```python
from build123d import *

# Parameters (mm, degrees)
SKETCH1_R                = 2.5
BOSS_EXTRUDE1_DEPTH      = 5
SKETCH3_W                = 20
SKETCH3_H                = 40
BOSS_EXTRUDE5_DEPTH      = 25
CUT_EXTRUDE2_DEPTH       = 75.20598847
CUT_EXTRUDE2_DEPTH_BACK  = 75.20598847
CUT_EXTRUDE_THIN13_DEPTH = 75.484252037
SKETCH8_W                = 5
SKETCH8_H                = 25
BOSS_EXTRUDE6_DEPTH      = 2
FILLET3_R                = 2
SKETCH9_W                = 5
SKETCH9_H                = 25
BOSS_EXTRUDE7_DEPTH      = 2
FILLET4_R                = 2
SKETCH11_R               = 4.5
CUT_EXTRUDE4_DEPTH       = 25
SKETCH12_R               = 6
SKETCH12_R_2             = 8
BOSS_EXTRUDE8_DEPTH      = 25
SKETCH13_R               = 2.5
CUT_EXTRUDE5_DEPTH       = 28
SKETCH14_R               = 4
CUT_EXTRUDE6_DEPTH       = 5
CUT_EXTRUDE7_DEPTH       = 18
CUT_EXTRUDE7_DEPTH_BACK  = 70
SKETCH15_R               = 2.5


with BuildPart() as part:
    # Sketch1 → Boss-Extrude1 (new body)
    with BuildSketch(Plane.XY):
        with BuildLine():
            Line((-33.639154819, 54.619565217), (6.360845181, 54.619565217))
            ThreePointArc((6.360845181, 54.619565217), (13.431912992, 51.690633029), (16.360845181, 44.619565217))
            Line((16.360845181, 44.619565217), (16.360845181, -5.380434783))
            ThreePointArc((16.360845181, -5.380434783), (13.431912992, -12.451502594), (6.360845181, -15.380434783))
            Line((6.360845181, -15.380434783), (-33.639154819, -15.380434783))
            ThreePointArc((-33.639154819, -15.380434783), (-40.710222631, -12.451502594), (-43.639154819, -5.380434783))
            Line((-43.639154819, -5.380434783), (-43.639154819, 44.619565217))
            ThreePointArc((-43.639154819, 44.619565217), (-40.710222631, 51.690633029), (-33.639154819, 54.619565217))
        make_face()
        with Locations((1.061250856, 48.159869042)):
            Circle(SKETCH1_R, mode=Mode.SUBTRACT)
        with Locations(Location((1.061250856, -9.840130958, 0), (0, 0, 180))):
            Circle(SKETCH1_R, mode=Mode.SUBTRACT)
        with Locations((-31.938749144, 19.159869042)):
            Circle(SKETCH1_R, mode=Mode.SUBTRACT)
    extrude(amount=BOSS_EXTRUDE1_DEPTH)

    # Sketch3 → Boss-Extrude5 (add)
    with BuildSketch(Plane.XY.offset(5)):
        Polygon((-24.438749144, 44.600432852), (-29.438749144, 44.600432852), (-29.438749144, 37.28199121), (-43.639154819, 37.28199121), (-43.639154819, 32.28199121), (-29.438749144, 32.28199121), (-29.438749144, 7.637328911), (-43.639154819, 7.637328911), (-43.639154819, 2.637328911), (-29.438749144, 2.637328911), (-29.438749144, -5.399567148), (-24.438749144, -5.399567148), (-24.438749144, -15.380434783), (-19.438749144, -15.380434783), (-19.438749144, -5.399567148), (-10.184597354, -5.399567148), (-10.184597354, -15.380434783), (-5.184597354, -15.380434783), (-5.184597354, -5.399567148), (0.561250856, -5.399567148), (0.561250856, 2.637328911), (14.825245568, 2.637328911), (14.825245568, 7.637328911), (0.561250856, 7.637328911), (0.561250856, 17.719700958), (14.825245568, 17.719700958), (14.825245568, 22.719700958), (0.561250856, 22.719700958), (0.561250856, 32.28199121), (14.825245568, 32.28199121), (14.825245568, 37.28199121), (0.561250856, 37.28199121), (0.561250856, 44.600432852), (-5.184597354, 44.600432852), (-5.184597354, 54.581300487), (-10.184597354, 54.581300487), (-10.184597354, 44.600432852), (-19.438749144, 44.600432852), (-19.438749144, 54.581300487), (-24.438749144, 54.581300487), align=None)
        with Locations((-14.438749144, 19.600432852)):
            Rectangle(SKETCH3_W, SKETCH3_H, mode=Mode.SUBTRACT)
    extrude(amount=BOSS_EXTRUDE5_DEPTH)

    # Sketch5 → Cut-Extrude2 (cut, two sides: drawn at the far end of the back side and taken through both)
    with BuildSketch(Plane.XZ.offset(-2.637328911).offset(-CUT_EXTRUDE2_DEPTH_BACK)):
        Polygon((-43.639154819, 30), (-43.639154819, 5), (-29.438749144, 30), align=None)
        Polygon((14.825245568, 30), (0.561250856, 30), (14.825245568, 5), align=None)
    extrude(amount=CUT_EXTRUDE2_DEPTH + CUT_EXTRUDE2_DEPTH_BACK, mode=Mode.SUBTRACT)

    # Sketch7 → Cut-Extrude-Thin13 (cut, through all)
    with BuildSketch(Plane.ZY.offset(24.438749144)):
        Polygon((30, 44.600432852), (5, 54.619565217), (8.72002984, 63.901880553), (33.72002984, 53.882748188), align=None)
        Polygon((5, -15.380434783), (30, -5.399567148), (33.707778838, -14.686782882), (8.707778838, -24.667650517), align=None)
    extrude(amount=-CUT_EXTRUDE_THIN13_DEPTH, mode=Mode.SUBTRACT)

    # Sketch8 → Boss-Extrude6 (add)
    with BuildSketch(Plane.XZ.offset(-39.600432852)):
        with Locations((-14.438749144, 17.5)):
            Rectangle(SKETCH8_W, SKETCH8_H)
    extrude(amount=BOSS_EXTRUDE6_DEPTH)

    # Fillet3
    fillet3_edges = [part.edges().sort_by_distance(p)[0] for p in [
        (-16.938749144, 37.600432852, 17.5),
        (-11.938749144, 37.600432852, 17.5),
    ]]
    fillet(fillet3_edges, radius=FILLET3_R - 0.0001)  # a hair under: the kernel refuses the full size

    # Sketch9 → Boss-Extrude7 (add)
    with BuildSketch(Plane(origin=(0, -0.399567148, 0), x_dir=(1, 0, 0), z_dir=(0, 1, 0))):
        with Locations((-14.690486301, -17.5)):
            Rectangle(SKETCH9_W, SKETCH9_H)
    extrude(amount=BOSS_EXTRUDE7_DEPTH)

    # Fillet4
    fillet4_edges = [part.edges().sort_by_distance(p)[0] for p in [
        (-12.190486301, 1.600432852, 17.5),
        (-17.190486301, 1.600432852, 17.5),
    ]]
    fillet(fillet4_edges, radius=FILLET4_R - 0.0001)  # a hair under: the kernel refuses the full size

    # Sketch11 → Cut-Extrude4 (cut)
    with BuildSketch(Plane.XY.offset(30)):
        with Locations((-31.938749144, 19.159869042)):
            Circle(SKETCH11_R)
    extrude(amount=-CUT_EXTRUDE4_DEPTH, mode=Mode.SUBTRACT)

    # Sketch12 → Boss-Extrude8 (add)
    with BuildSketch(Plane.XY.offset(5)):
        with Locations((1.061250856, 48.159869042)):
            Circle(SKETCH12_R)
        with Locations((1.061250856, -9.840130958)):
            Circle(SKETCH12_R)
        with Locations((-31.938749144, 19.159869042)):
            Circle(SKETCH12_R_2)
    extrude(amount=BOSS_EXTRUDE8_DEPTH)

    # Sketch13 → Cut-Extrude5 (cut)
    with BuildSketch(Plane(origin=(0, 0, 0), x_dir=(-1, 0, 0), z_dir=(0, 0, -1))):
        with Locations((31.938749144, 19.159869042)):
            Circle(SKETCH13_R)
        with Locations((-1.061250856, -9.840130958)):
            Circle(SKETCH13_R)
        with Locations((-1.061250856, 48.159869042)):
            Circle(SKETCH13_R)
    extrude(amount=-CUT_EXTRUDE5_DEPTH, mode=Mode.SUBTRACT)

    # Sketch14 → Cut-Extrude6 (cut)
    with BuildSketch(Plane.XY.offset(30)):
        with Locations((-31.938749144, 19.159869042)):
            Circle(SKETCH14_R)
        with Locations((1.061250856, 48.159869042)):
            Circle(SKETCH14_R)
        with Locations((1.061250856, -9.840130958)):
            Circle(SKETCH14_R)
    extrude(amount=-CUT_EXTRUDE6_DEPTH, mode=Mode.SUBTRACT)

    # Sketch15 → Cut-Extrude7 (cut, two sides: drawn at the far end of the back side and taken through both)
    with BuildSketch(Plane(origin=(0, 44.600432852, 0), x_dir=(1, 0, 0), z_dir=(0, 1, 0)).offset(-CUT_EXTRUDE7_DEPTH_BACK)):
        with Locations(Location((-14.811673249, -17.5, 0), (0, 0, 75.612724185))):
            Circle(SKETCH15_R)
    extrude(amount=CUT_EXTRUDE7_DEPTH + CUT_EXTRUDE7_DEPTH_BACK, mode=Mode.SUBTRACT)


solid = part.part
```
The listing builds one solid part. Answer for the finished solid, in the listing's coordinates (mm). A direction names the side the tool comes from. Give positions to 0.01 mm unless a question says otherwise; leave off trailing zeros. Order: outer loops, then holes, each group sorted by start corner. A loop starts at its lowest first (then second) coordinate and runs counter-clockwise, first axis right, second up. Notation, with made-up numbers: M 8,85.5 L 39,85.5 A4 cw 39,90.5 Z; hole C 87.25,78.5 d10. An arc over 180 degrees is marked long. Put each result on its own line as item: value. Start each with the question number.
Item 1: The part is cut by section C-C, the plane y = 49. Determine the outline of the cut face in (x, z), and give its area (3 significant figures).
Item 2: Which of the six approach directions +Z, -Z, +X, -X, +Y, -Y give full straight-line access (tool end or side, diameter ignored) to faces 4 (the face through (-29.439, -1, 17)), 5 (the face through (-27, 44.6, 17)), 6 (the face through (-21, -0.4, 17)), 7 (the face through (-19.439, 48, 15))?
Item 3: Find the intervals of material crossed by line 1 along Y through (x, z) = (-31.5, 21); line 2 along Y through (x, z) = (-11.5, 26.5); line 3 along Z through (x, y) = (-29, -9.5), in increasing order.
Item 4: Flat-ended cylindrical pins translate along their axes: P1, Ø5, axis at x = 10, z = 16, coming from the -Y side; P2, Ø6, axis at x = -12, y = 37.5, coming from the -Z side; P3, Ø10.5, axis at y = 28.5, z = 20.5, coming from the +X side; P4, Ø2, axis at x = -35.5, z = 24.5, coming from the -Y side. Find the tip coordinate at first contact, or state that the pin passes through.
Item 5: The part is cut by section B-B, the plane z = 4. Determine the outline of the cut face in (x, y), and give its area (3 significant figures).
Item 6: The part is cut by section D-D, the plane y = 36.5. Determine the outline of the cut face in (x, z), and give its area (3 significant figures).
Item 7: For a pull along Z with two mould halves and no side action, classify faces 1 (the face through (-1, -12, 25)), 2 (the face through (-12.377, 41.051, 16.934)), 3 (the face through (0.561, 13, 17)) as +Z half, -Z half, draft (parallel to the pull), parting line (faces both ways), or undercut.
Answer key:
1. outline: M -42.63,0 L -1.29,0 L -1.29,25 L -2.85,25 L -2.85,30 L -4.88,30 L -4.88,5 L -5.18,5 L -5.18,19.02 L -10.18,19.02 L -10.18,5 L -19.44,5 L -19.44,19.02 L -24.44,19.02 L -24.44,5 L -42.63,5 Z; M 3.42,0 L 15.35,0 L 15.35,5 L 7,5 L 7,30 L 4.97,30 L 4.97,25 L 3.42,25 Z
1. area: 570 mm²
2. face 4: +Z, -X, -Y
2. face 5: +Z, -X, +Y
2. face 6: +Z
2. face 7: +Z, +Y
3. line 1: y = 2.64 to 7.64, 11.17 to 16.7, 21.62 to 27.15, 32.28 to 37.28
3. line 2: y = -5.4 to -0.4, 39.6 to 44.6
3. line 3: z = 0 to 5
4. P1: stops at y = 2.64
4. P2: stops at z = 0
4. P3: stops at x = 8.06
4. P4: stops at y = 11.58
5. outline: M -43.64,-5.38 A10 ccw -33.64,-15.38 L 6.36,-15.38 A10 ccw 16.36,-5.38 L 16.36,44.62 A10 ccw 6.36,54.62 L -33.64,54.62 A10 ccw -43.64,44.62 Z; hole C -31.94,19.16 d5; hole C 1.06,-9.84 d5; hole C 1.06,48.16 d5
5. area: 4,060 mm²
6. outline: M -43.64,0 L 16.36,0 L 16.36,5 L 14.83,5 L 0.56,30 L -4.44,30 L -4.44,5 L -24.44,5 L -24.44,30 L -29.44,30 L -43.64,5 Z
6. area: 906 mm²
7. face 1: +Z half
7. face 2: undercut
7. face 3: draft
